For this review, use the dimensioned drawing (mm, ordinates from the lowest corner) and the shaded views. Give positions to 0.01 mm unless a question says otherwise; leave off trailing zeros. Order: outer loops, then holes, each group sorted by start corner. A loop starts at its lowest first (then second) coordinate and runs counter-clockwise, first axis right, second up.
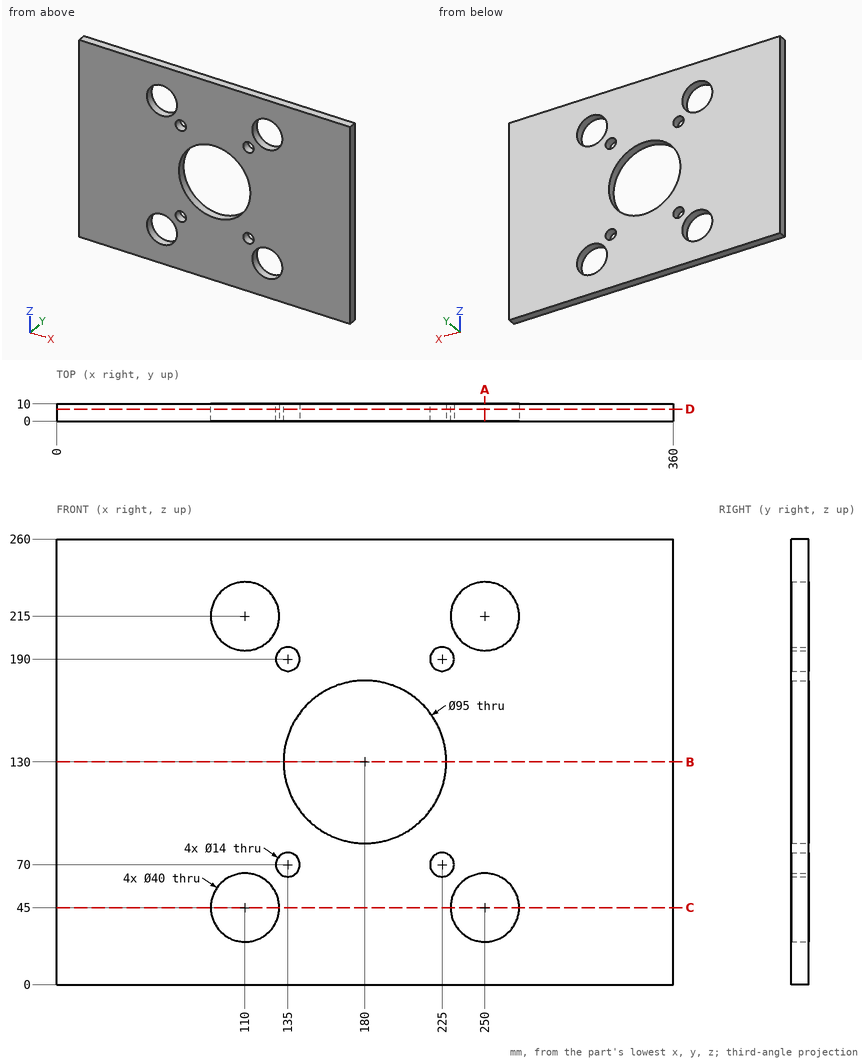
1. Take a section at D-D (y = 7). State how many separate pieces and enclosed holes the cut face has, then the cut area to 3 significant figures.
Recorded:
separate pieces: 1
enclosed holes: 9
area: 80,900 mm2
2. For line 1 along Z through (x, y) = (250, 7.5); line 2 along X through (y, z) = (8.75, 203.5); line 3 along X through (y, z) = (5.75, 38) (3 decimals), list the stretches that pass through material, from the lowest coordinate up.
Recorded:
line 1: z = 0 to 25, 65 to 195, 235 to 260
line 2: x = 0 to 93.64, 126.36 to 233.64, 266.36 to 360
line 3: x = 0 to 91.265, 128.735 to 231.265, 268.735 to 360
3. For pin 1 (3 mm diameter, centred on x = 114.5, y = 7.5, fed in from -Z), flat-tipped, find the tip position at first contact; note if it passes through.
Recorded:
pin 1: stops at z = 0
4. Take a section at C-C (z = 45). State the section outline as (x, y) points.
Recorded:
outline: (0, 0) - (90, 0) - (90, 10) - (0, 10) - close; (130, 0) - (230, 0) - (230, 10) - (130, 10) - close; (270, 0) - (360, 0) - (360, 10) - (270, 10) - close
5. Take a section at B-B (z = 130). State the section outline as (x, y) points, then the cut area to 3 significant figures.
Recorded:
outline: (0, 0) - (132.5, 0) - (132.5, 10) - (0, 10) - close; (227.5, 0) - (360, 0) - (360, 10) - (227.5, 10) - close
area: 2,650 mm2
6. Take a section at A-A (x = 250). State the section outline as (y, z) points, then the cut area to 3 significant figures.
Recorded:
outline: (0, 0) - (10, 0) - (10, 25) - (0, 25) - close; (0, 65) - (10, 65) - (10, 195) - (0, 195) - close; (0, 235) - (10, 235) - (10, 260) - (0, 260) - close
area: 1,800 mm2
